Input: dimensioned drawing with shaded views. Units: mm. Origin: part minimum x, y, z. Coordinates: 2 decimals unless noted, no trailing zeros. Order: outer loops, then holes, each group sorted by start corner. A loop starts at its lowest first (then second) coordinate and runs counter-clockwise, first axis right, second up.
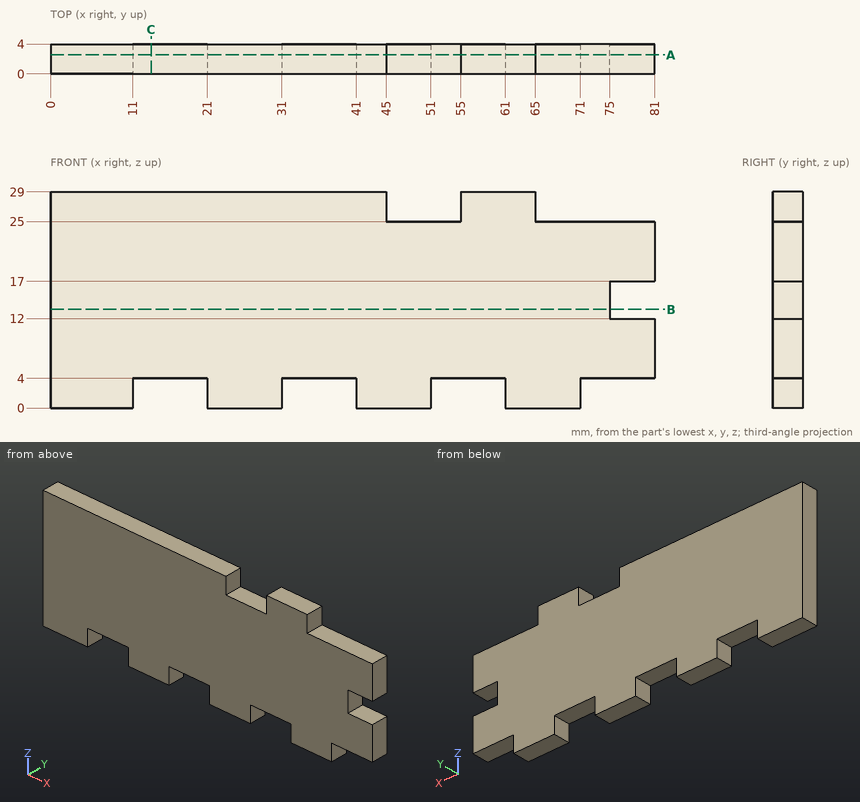
1. Material intervals for line 1 along X through (y, z) = (2.7, 2.5); line 2 along Z through (x, y) = (76, 3.5); line 3 along X through (y, z) = (3.4, 27), sorted ascending.
2. Section query A-A, the plane y = 2.55. Output: boundary loops of the cut face in (x, z), plus the area to 4 significant figures.
3. Section query B-B, the plane z = 13.25. Output: boundary loops of the cut face in (x, y), plus the area to 3 significant figures.
4. Section query C-C, the plane x = 13.5. Output: boundary loops of the cut face in (y, z).
5. Contact query for flat-ended pins moving along their axis: P1, Ø2, axis at x = 76.5, y = 2, coming from the -Z side; P2, Ø1.2, axis at y = 1.5, z = 2.5, coming from the +X side; P3, Ø1.2, axis at y = 2.5, z = 28, coming from the +X side. Output: stop coordinate, or through.
Answer key:
1. line 1: x = 0 to 11, 21 to 31, 41 to 51, 61 to 71
1. line 2: z = 4 to 12, 17 to 25
1. line 3: x = 0 to 45, 55 to 65
2. outline: (0, 0) - (11, 0) - (11, 4) - (21, 4) - (21, 0) - (31, 0) - (31, 4) - (41, 4) - (41, 0) - (51, 0) - (51, 4) - (61, 4) - (61, 0) - (71, 0) - (71, 4) - (81, 4) - (81, 12) - (75, 12) - (75, 17) - (81, 17) - (81, 25) - (65, 25) - (65, 29) - (55, 29) - (55, 25) - (45, 25) - (45, 29) - (0, 29) - close
2. area: 2,055 mm2
3. outline: (0, 0) - (75, 0) - (75, 4) - (0, 4) - close
3. area: 300 mm2
4. outline: (0, 4) - (4, 4) - (4, 29) - (0, 29) - close
5. P1: stops at z = 4
5. P2: stops at x = 71
5. P3: stops at x = 65
